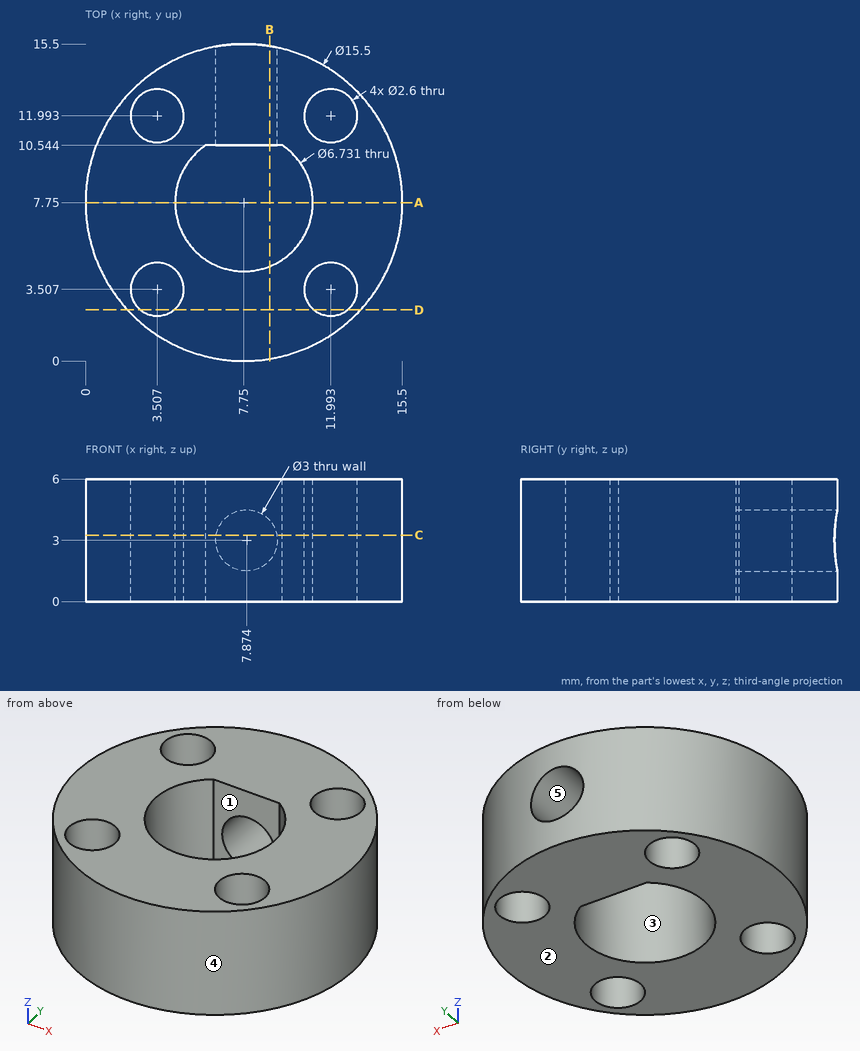
Geometry: see drawing. Coordinates: mm, zero at the bounding-box minimum. A direction names the side the tool comes from. Round coordinates to 2 decimals unless told otherwise and drop trailing zeros. Write each loop counter-clockwise with the first axis right and the second up, starting at its lowest first coordinate (ties: lowest second). Pieces come first, ordered by that corner, then holes.
1) Ray query, L1, parallel to X at y = 12.5, z = 4.25 (1 decimal); L2, parallel to X at y = 9.25, z = 1.25 (1 decimal); L3, parallel to Y at x = 5.5, z = 3.75 (1 decimal). Return the intervals inside material, ascending.
2) Reachability of the marked faces 1 and 2 from +Z, -Z, +X, -X, +Y, -Y: full face, straight path, thin tool, end or side. Return the list, or none.
3) Draft query along Y for the marked faces 3, 4 and 5. Return one class per face: pulls with the +Y half, pulls with the -Y half, needs draft (parallel to the pull), parting line crosses it, or undercut.
4) Cut plane D-D (y = 2.5). Return the cut outline in (x, z) (1 decimal).
5) Cut plane C-C (z = 3.25). Count the separate pieces of the cut face and the enclosed holes in it, then the cut area to 3 significant figures.
6) Contact query for a flat-ended pin moving along its axis: P1, Ø1, axis at y = 6, z = 3.5, coming from the -X side. Output: stop coordinate, or through.
7) Cut plane A-A (y = 7.75). Return the cut outline in (x, z) (1 decimal), then the cut area to 3 significant figures.
8) Cut plane B-B (x = 9). Return the cut outline in (y, z) (1 decimal).
Geometry says:
1. L1: x = 1.6 to 2.3, 4.7 to 7, 8.7 to 10.8, 13.2 to 13.9
1. L2: x = 0.1 to 4.7, 10.8 to 15.4
1. L3: y = 0.3 to 5.2, 10.3 to 15.2
2. face 1: +Z, -Z
2. face 2: -Z, +X, -X, +Y, -Y
3. face 3: undercut
3. face 4: parting line crosses it
3. face 5: needs draft
4. outline: (2, 0) - (2.7, 0) - (2.7, 6) - (2, 6) - close; (4.3, 0) - (11.2, 0) - (11.2, 6) - (4.3, 6) - close; (12.8, 0) - (13.5, 0) - (13.5, 6) - (12.8, 6) - close
5. separate pieces: 1
5. enclosed holes: 4
5. area: 119 mm2
6. P1: stops at x = 0.1
7. outline: (0, 0) - (4.4, 0) - (4.4, 6) - (0, 6) - close; (11.1, 0) - (15.5, 0) - (15.5, 6) - (11.1, 6) - close
7. area: 52.6 mm2
8. outline: (0.1, 0) - (4.6, 0) - (4.6, 6) - (0.1, 6) - close; (10.5, 0) - (15.4, 0) - (15.4, 2) - (10.5, 2) - close; (10.5, 4) - (15.4, 4) - (15.4, 6) - (10.5, 6) - close
